Verification items for the finished model (mm, model axes). Face numbers are marked on the shaded views. A direction names the side the tool comes from. Round coordinates to 2 decimals unless told otherwise and drop trailing zeros. Order: outer loops, then holes, each group sorted by start corner. A loop starts at its lowest first (then second) coordinate and runs counter-clockwise, first axis right, second up. Notation, with made-up numbers: M 23.25,13 L 58.25,13 A21 cw 58.25,31 Z; hole C 83.25,17 d1. An arc over 180 degrees is marked long. Use CSV: the item, a comma, the result in double quotes. Start each with the question number.
Q1. Sectioned sample at B-B (x = 14). Enter the section's corners in (y, z), and give its area (3 significant figures).
Q2. Sectioned sample at A-A (z = 13.5). Enter the section's corners in (x, y).
Q3. Sectioned sample at C-C (y = 20.5). Enter the section's corners in (x, z), and give its area (3 significant figures).
Q4. Gauge pin test, flat ends, axial feed: pin 1 Ø10 at (y, z) = (18, 12.5) entering from +X; pin 2 Ø6.5 at (x, z) = (19, 15.5) entering from +Y; pin 3 Ø8 at (y, z) = (7, 19) entering from +X; pin 4 Ø10 at (x, y) = (19, 20.5) entering from +Z. Record the tip position at first contact, or that the pin passes through.
Q5. Sectioned sample at D-D (x = 18.5). Enter the section's corners in (y, z).
Q6. Scan lines: line 1 (Z direction, x = 13.5, y = 15); line 2 (Z direction, x = 12, y = 4); line 3 (X direction, y = 17, z = 13). Record each from-to range of solid material in increasing order.
Q7. Set-up check for the marked faces 1, 2, 3, 4 and 5: record each of +Z, -Z, +X, -X, +Y, -Y from which the full face is reachable in a straight line by a thin tool's end or side.
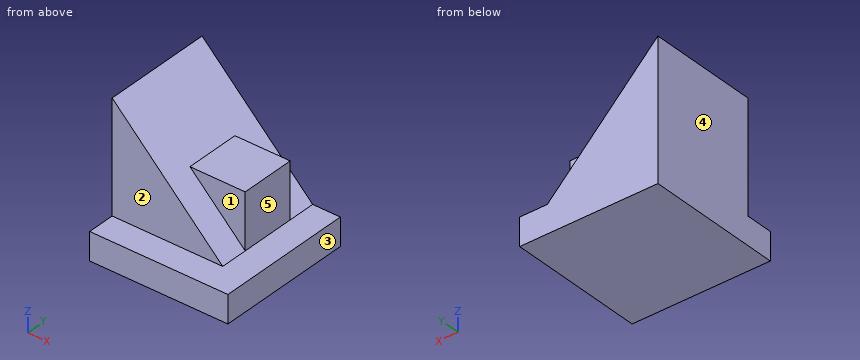
```python
from build123d import *

# Parameters (mm, degrees)
F0_W     = 31.75
F0_H     = 31.75
F1_DEPTH = 6.35
F3_DEPTH = 25.4
F5_DEPTH = 19.05
F7_DEPTH = 6.35


with BuildPart() as f1:
    # F0 (on Top) → F1 (new body)
    with BuildSketch(Plane.XY):
        with Locations((15.875, 15.875)):
            Rectangle(F0_W, F0_H)
    extrude(amount=F1_DEPTH)

    # F2 (on face) → F3 (join)
    with BuildSketch(Plane(origin=(0, 31.75, 0), x_dir=(-1, 0, 0), z_dir=(0, 1, 0))):
        Polygon((-25.4, 6.35), (0, 6.35), (0, 31.75), align=None)
    extrude(amount=-F3_DEPTH)

    # F4 (on face) → F5 (join)
    with BuildSketch(Plane(origin=(0, 31.75, 0), x_dir=(-1, 0, 0), z_dir=(0, 1, 0))):
        Polygon((-25.4, 19.05), (-25.4, 6.35), (-12.7, 19.05), align=None)
    extrude(amount=-F5_DEPTH)

    # F6 (on face) → F7 (cut)
    with BuildSketch(Plane(origin=(0, 31.75, 0), x_dir=(-1, 0, 0), z_dir=(0, 1, 0))):
        Polygon((-25.4, 19.05), (-25.4, 6.35), (-12.7, 19.05), align=None)
    extrude(amount=-F7_DEPTH, mode=Mode.SUBTRACT)


solid = f1.part
```
Verdict:
1,outline,"M 0,0 L 31.75,0 L 31.75,17.75 L 25.4,17.75 L 25.4,19.05 L 12.7,19.05 L 12.7,17.75 L 6.35,17.75 L 6.35,6.35 L 0,6.35 Z"
1,area,"508 mm²"
2,outline,"M 0,6.35 L 18.25,6.35 L 18.25,12.7 L 25.4,12.7 L 25.4,25.4 L 18.25,25.4 L 18.25,31.75 L 0,31.75 Z"
3,outline,"M 0,0 L 31.75,0 L 31.75,6.35 L 25.4,6.35 L 25.4,19.05 L 12.7,19.05 L 0,31.75 Z"
3,area,"605 mm²"
4,pin 1,"stops at x = 25.4"
4,pin 2,"stops at y = 31.75"
4,pin 3,"stops at x = 16.75"
4,pin 4,"stops at z = 19.05"
5,outline,"M 0,0 L 31.75,0 L 31.75,13.25 L 25.4,13.25 L 25.4,19.05 L 12.7,19.05 L 12.7,13.25 L 6.35,13.25 L 6.35,6.35 L 0,6.35 Z"
6,line 1,"z = 0 to 19.05"
6,line 2,"z = 0 to 6.35"
6,line 3,"x = 0 to 25.4"
7,face 1,"+Z, +X, -Y"
7,face 2,"+Z, +X, -X, -Y"
7,face 3,"+Z, -Z, +X, +Y, -Y"
7,face 4,"+Z, -Z, -X, +Y, -Y"
7,face 5,"+Z, +X, +Y, -Y"
